Geometry: final body of the model. Coordinates: model frame, mm. Face numbers are marked on the shaded views. A direction names the side the tool comes from. Round coordinates to 2 decimals unless told otherwise and drop trailing zeros. Loops run counter-clockwise (first coordinate to the right, second up) from the corner with the lowest first, then second, coordinate; pieces in that order, holes last. Notation, with made-up numbers: (29, -31) -> (40, -31) arc R32 ccw to (40, -1) -> close; hole circle Ø9 at (-29.5, 12). An arc over 180 degrees is marked (long way). Answer in a Markdown table with one row per item.
```python
from build123d import *

# Parameters (mm, degrees)
SKIZZE1_W                       = 124
SKIZZE1_H                       = 57
AUFSATZ_LINEAR_AUSTRAGEN1_DEPTH = 25
SKIZZE2_W                       = 8
SKIZZE2_H                       = 8
SCHNITT_LINEAR_AUSTRAGEN4_DEPTH = 18
SKIZZE5_W                       = 120
SKIZZE5_H                       = 20
SKIZZE5_W_2                     = 105
SKIZZE5_H_2                     = 13
SCHNITT_LINEAR_AUSTRAGEN5_DEPTH = 23
SKIZZE6_R                       = 14
SKIZZE6_W                       = 31
SKIZZE6_H                       = 7.5
SCHNITT_LINEAR_AUSTRAGEN6_DEPTH = 2


with BuildPart() as part:
    # Skizze1 → Aufsatz-Linear austragen1 (new body)
    with BuildSketch(Plane.XY):
        with Locations((-40.959148289, 0.914772727)):
            Rectangle(SKIZZE1_W, SKIZZE1_H)
    extrude(amount=AUFSATZ_LINEAR_AUSTRAGEN1_DEPTH)

    # Skizze2 → Schnitt-Linear austragen4 (cut)
    with BuildSketch(Plane.XY.offset(25)):
        with Locations((17.040851711, 0.914772727)):
            Rectangle(SKIZZE2_W, SKIZZE2_H)
        with Locations((-98.959148289, 0.914772727)):
            Rectangle(SKIZZE2_W, SKIZZE2_H)
    extrude(amount=-SCHNITT_LINEAR_AUSTRAGEN4_DEPTH, mode=Mode.SUBTRACT)

    # Skizze5 → Schnitt-Linear austragen5 (cut)
    with BuildSketch(Plane(origin=(0, 0, 0), x_dir=(-1, 0, 0), z_dir=(0, 0, -1))):
        with Locations((40.959148289, 17.414772727)):
            Rectangle(SKIZZE5_W, SKIZZE5_H)
        with Locations((40.959148289, 0.914772727)):
            Rectangle(SKIZZE5_W_2, SKIZZE5_H_2)
        with Locations((40.959148289, -15.585227273)):
            Rectangle(SKIZZE5_W, SKIZZE5_H)
    extrude(amount=-SCHNITT_LINEAR_AUSTRAGEN5_DEPTH, mode=Mode.SUBTRACT)

    # Skizze6 → Schnitt-Linear austragen6 (cut)
    with BuildSketch(Plane(origin=(0, 29.414772727, 0), x_dir=(1, 0, 0), z_dir=(0, 1, 0))):
        with Locations((-2.959148289, 0)):
            Circle(SKIZZE6_R)
        with Locations((-78.959148289, 0)):
            Circle(SKIZZE6_R)
        with Locations((-40.959148289, -3.75)):
            Rectangle(SKIZZE6_W, SKIZZE6_H)
    extrude(amount=-SCHNITT_LINEAR_AUSTRAGEN6_DEPTH, mode=Mode.SUBTRACT)


solid = part.part
```
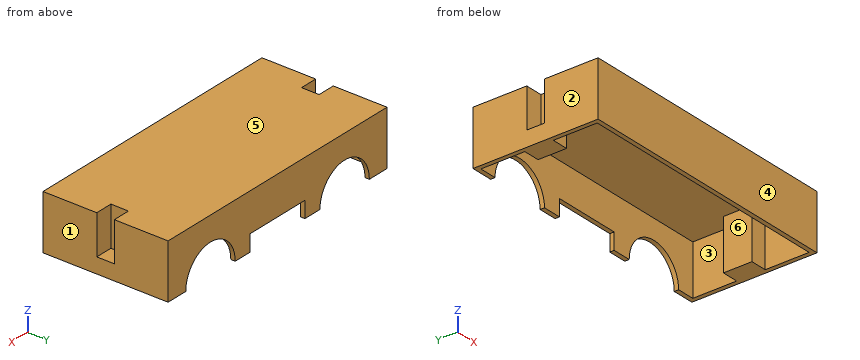
Item 1: First-contact query: P1, Ø2.5, axis at y = 2.5, z = 14.5, coming from the -X side; P2, Ø8, axis at x = -31.5, y = 6.5, coming from the -Z side; P3, Ø12, axis at x = -73, z = 5, coming from the +Y side. Flat tips, straight axial feed; report the tip coordinate or a pass-through.
Ans:
| item | result |
|---|---|
| P1 | x = -94.96 |
| P2 | z = 23 |
| P3 | y = -25.59 |
Item 2: Section query A-A, the plane x = -44. Output: boundary loops of the cut face in (y, z).
Ans:
| item | result |
|---|---|
| outline | (-27.59, 0) -> (-25.59, 0) -> (-25.59, 23) -> (27.41, 23) -> (27.41, 7.5) -> (29.41, 7.5) -> (29.41, 25) -> (-27.59, 25) -> close |
Item 3: Ray query, L1, parallel to Y at x = 15, z = 18.5; L2, parallel to X at y = 20, z = 10.5; L3, parallel to Y at x = -69, z = 10.5. Return the intervals inside material, ascending.
Ans:
| item | result |
|---|---|
| L1 | -27.59 to -25.59, -5.59 to -3.09, 4.91 to 7.41, 27.41 to 29.41 |
| L2 | -102.96 to -100.96, 19.04 to 21.04 |
| L3 | -27.59 to -25.59, 27.41 to 29.41 |
Item 4: Mould query, pull axis X, two halves, no side actions, for the marked faces 1, 2, 3 and 4. Classes: released by +X, released by -X, zero draft, split by the parting line, or undercut.
Ans:
| item | result |
|---|---|
| face 1 | released by +X |
| face 2 | released by -X |
| face 3 | undercut |
| face 4 | zero draft |
Item 5: Section query D-D, the plane y = 10.5. Output: boundary loops of the cut face in (x, z), and give its area (3 significant figures).
Ans:
| item | result |
|---|---|
| outline | (-102.96, 0) -> (-100.96, 0) -> (-100.96, 23) -> (19.04, 23) -> (19.04, 0) -> (21.04, 0) -> (21.04, 25) -> (-102.96, 25) -> close |
| area | 340 mm2 |
Item 6: Set-up query: the marked faces 5 and 6. Return all of +Z, -Z, +X, -X, +Y, -Y with unobstructed straight access to the full face (end or side cutting, diameter ignored); none if empty.
Ans:
| item | result |
|---|---|
| face 5 | +Z, +X, -X, +Y, -Y |
| face 6 | -Z |
Item 7: Section query B-B, the plane z = 16.25. Output: boundary loops of the cut face in (x, y).
Ans:
| item | result |
|---|---|
| outline | (-102.96, -27.59) -> (21.04, -27.59) -> (21.04, -3.09) -> (13.04, -3.09) -> (13.04, 4.91) -> (21.04, 4.91) -> (21.04, 29.41) -> (-102.96, 29.41) -> (-102.96, 4.91) -> (-94.96, 4.91) -> (-94.96, -3.09) -> (-102.96, -3.09) -> close; hole (-100.96, -25.59) -> (19.04, -25.59) -> (19.04, -5.59) -> (11.54, -5.59) -> (11.54, 7.41) -> (19.04, 7.41) -> (19.04, 27.41) -> (-100.96, 27.41) -> (-100.96, 7.41) -> (-93.46, 7.41) -> (-93.46, -5.59) -> (-100.96, -5.59) -> close |
